```python
from build123d import *

# Parameters (mm, degrees)
CROQUIS1_R                      = 1.625
SALIENTE_EXTRUIR1_DEPTH         = 4
CORTAR_EXTRUIR1_START           = -190
CORTAR_EXTRUIR1_DEPTH           = 190
CROQUIS4_R                      = 3.35997123
CORTAR_EXTRUIR2_DEPTH           = 1.8
CORTAR_EXTRUIR2_DRAFT           = -44
CORTAR_EXTRUIR2_PROFILE_2_DEPTH = 1.8
CORTAR_EXTRUIR2_PROFILE_2_DRAFT = -44
CORTAR_EXTRUIR2_PROFILE_3_DEPTH = 1.8
CORTAR_EXTRUIR2_PROFILE_3_DRAFT = -44
CORTAR_EXTRUIR2_PROFILE_4_DEPTH = 1.8
CORTAR_EXTRUIR2_PROFILE_4_DRAFT = -44
CORTAR_EXTRUIR3_DEPTH           = 2
CROQUIS9_W                      = 0.961538462
CROQUIS9_H                      = 7.5
CORTAR_EXTRUIR5_DEPTH           = 1.5


with BuildPart() as part:
    # Croquis1 → Saliente-Extruir1 (new body)
    with BuildSketch(Plane.XY):
        Polygon((-32.320991683, -51.284123552), (-32.320991683, 29.135238548), (157.679008317, 29.135238548), (157.679008317, -51.284123552), (105.737585684, -51.284123552), (105.737585684, -25.284123552), (45.737585684, -25.284123552), (45.737585684, -51.284123552), align=None)
        with Locations((23.679008317, 21.135238548)):
            Circle(CROQUIS1_R, mode=Mode.SUBTRACT)
        with Locations((101.679008317, 21.135238548)):
            Circle(CROQUIS1_R, mode=Mode.SUBTRACT)
        with Locations((-25.720991683, -43.884123552)):
            Circle(CROQUIS1_R, mode=Mode.SUBTRACT)
        with Locations((151.079008317, -44.084123552)):
            Circle(CROQUIS1_R, mode=Mode.SUBTRACT)
    extrude(amount=SALIENTE_EXTRUIR1_DEPTH)

    # Croquis3 → Cortar-Extruir1 (cut)
    with BuildSketch(Plane(origin=(157.679008317, 0, 0), x_dir=(0, 0, -1), z_dir=(1, 0, 0)).offset(CORTAR_EXTRUIR1_START)):
        Polygon((-4, 29.135238548), (0, 29.135238548), (-4, 27.880003721), align=None)
    extrude(amount=CORTAR_EXTRUIR1_DEPTH, mode=Mode.SUBTRACT)


with BuildPart() as cortar_extruir2_tool:
    # Croquis4 → Cortar-Extruir2 (with draft: the straight prism first)
    with BuildSketch(Plane.XY.offset(4)):
        with Locations((23.679008317, 21.135238548)):
            Circle(CROQUIS4_R)
    extrude(amount=-CORTAR_EXTRUIR2_DEPTH)
    # Cortar-Extruir2: the draft: its side faces are tilted about the plane it starts from
    cortar_extruir2_sides = [cortar_extruir2_tool.faces().sort_by_distance(p)[0] for p in [
        (20.319037087, 21.135238548, 3.1),
    ]]
    draft(cortar_extruir2_sides, Plane.XY.offset(4), CORTAR_EXTRUIR2_DRAFT)


with BuildPart() as part_1:
    add(part.part)

    # Cortar-Extruir2: cut by cortar_extruir2_tool
    add(cortar_extruir2_tool.part, mode=Mode.SUBTRACT)


with BuildPart() as cortar_extruir2_profile_2_tool:
    # Croquis4 → Cortar-Extruir2 profile 2 (with draft: the straight prism first)
    with BuildSketch(Plane.XY.offset(4)):
        with Locations((101.679008317, 21.135238548)):
            Circle(CROQUIS4_R)
    extrude(amount=-CORTAR_EXTRUIR2_PROFILE_2_DEPTH)
    # Cortar-Extruir2 profile 2: the draft: its side faces are tilted about the plane it starts from
    cortar_extruir2_profile_2_sides = [cortar_extruir2_profile_2_tool.faces().sort_by_distance(p)[0] for p in [
        (98.319037087, 21.135238548, 3.1),
    ]]
    draft(cortar_extruir2_profile_2_sides, Plane.XY.offset(4), CORTAR_EXTRUIR2_PROFILE_2_DRAFT)


with BuildPart() as part_2:
    add(part_1.part)

    # Cortar-Extruir2 profile 2: cut by cortar_extruir2_profile_2_tool
    add(cortar_extruir2_profile_2_tool.part, mode=Mode.SUBTRACT)


with BuildPart() as cortar_extruir2_profile_3_tool:
    # Croquis4 → Cortar-Extruir2 profile 3 (with draft: the straight prism first)
    with BuildSketch(Plane.XY.offset(4)):
        with Locations((-25.720991683, -43.884123552)):
            Circle(CROQUIS4_R)
    extrude(amount=-CORTAR_EXTRUIR2_PROFILE_3_DEPTH)
    # Cortar-Extruir2 profile 3: the draft: its side faces are tilted about the plane it starts from
    cortar_extruir2_profile_3_sides = [cortar_extruir2_profile_3_tool.faces().sort_by_distance(p)[0] for p in [
        (-29.080962913, -43.884123552, 3.1),
    ]]
    draft(cortar_extruir2_profile_3_sides, Plane.XY.offset(4), CORTAR_EXTRUIR2_PROFILE_3_DRAFT)


with BuildPart() as part_3:
    add(part_2.part)

    # Cortar-Extruir2 profile 3: cut by cortar_extruir2_profile_3_tool
    add(cortar_extruir2_profile_3_tool.part, mode=Mode.SUBTRACT)


with BuildPart() as cortar_extruir2_profile_4_tool:
    # Croquis4 → Cortar-Extruir2 profile 4 (with draft: the straight prism first)
    with BuildSketch(Plane.XY.offset(4)):
        with Locations((151.079008317, -44.084123552)):
            Circle(CROQUIS4_R)
    extrude(amount=-CORTAR_EXTRUIR2_PROFILE_4_DEPTH)
    # Cortar-Extruir2 profile 4: the draft: its side faces are tilted about the plane it starts from
    cortar_extruir2_profile_4_sides = [cortar_extruir2_profile_4_tool.faces().sort_by_distance(p)[0] for p in [
        (147.719037087, -44.084123552, 3.1),
    ]]
    draft(cortar_extruir2_profile_4_sides, Plane.XY.offset(4), CORTAR_EXTRUIR2_PROFILE_4_DRAFT)


with BuildPart() as part_4:
    add(part_3.part)

    # Cortar-Extruir2 profile 4: cut by cortar_extruir2_profile_4_tool
    add(cortar_extruir2_profile_4_tool.part, mode=Mode.SUBTRACT)

    # Croquis6 → Cortar-Extruir3 (cut)
    with BuildSketch(Plane.XY.offset(4)):
        Polygon((16.032465101, -18.974654774), (-1.066430914, -18.974654774), (-6.350280368, -35.236671251), (-11.634129822, -18.974654774), (-28.733025837, -18.974654774), (-14.899728375, -8.924175866), (-20.183577829, 7.337840611), (-6.350280368, -2.712638297), (7.483017094, 7.337840611), (2.19916764, -8.924175866), align=None)
        Polygon((109.325551533, -18.974654774), (126.424447548, -18.974654774), (131.708297002, -35.236671251), (136.992146456, -18.974654774), (154.091042471, -18.974654774), (140.25774501, -8.924175866), (145.541594464, 7.337840611), (131.708297002, -2.712638297), (117.874999541, 7.337840611), (123.158848995, -8.924175866), align=None)
    extrude(amount=-CORTAR_EXTRUIR3_DEPTH, mode=Mode.SUBTRACT)

    # Croquis9 → Cortar-Extruir5 (cut)
    # profile 1 of 7: a face of its own
    with BuildSketch(Plane.XY.offset(4)):
        Polygon((84.938623702, -0.162159389), (83.97708524, -0.162159389), (83.97708524, 2.546674746), (80.24661649, -0.162159389), (78.832854471, -0.162159389), (83.464765529, 3.203225226), (78.448239086, 7.337840611), (79.771856875, 7.337840611), (83.97708524, 3.871794938), (83.97708524, 7.337840611), (84.938623702, 7.337840611), align=None)
    # profile 2 of 7: a face of its own
    with BuildSketch(Plane.XY.offset(4)):
        Polygon((73.111700625, -0.162159389), (68.688623702, 7.337840611), (69.747818413, 7.337840611), (71.166087644, 4.933994457), (75.309717452, 4.933994457), (76.759537163, 7.337840611), (77.823239086, 7.337840611), (73.304008317, -0.162159389), align=None)
        Polygon((73.21536649, 1.457431957), (74.846977067, 4.164763688), (71.618311202, 4.164763688), align=None, mode=Mode.SUBTRACT)
    # profile 3 of 7: a face of its own
    with BuildSketch(Plane.XY.offset(4)):
        with Locations((66.861700625, 3.587840611)):
            Rectangle(CROQUIS9_W, CROQUIS9_H)
    # profile 4 of 7: a face of its own
    with BuildSketch(Plane.XY.offset(4)):
        with BuildLine():
            Line((64.361700625, -0.162159389), (62.432614086, -0.162159389))
            add(Edge.make_bspline(
                [(62.432614086, -0.162159389), (62.303407857, -0.161829936), (62.056004322, -0.161199101), (61.701380518, -0.157593434), (61.379408986, -0.147395372), (61.089802811, -0.138594846), (60.832957985, -0.122524062), (60.608382947, -0.107262614), (60.416359573, -0.087004293), (60.299642276, -0.06843303), (60.24661649, -0.059995928)],
                knots=[0, 0, 0, 0, 1.415751681, 2.71087525, 3.885633551, 4.945392006, 5.885335126, 6.705178082, 7.411750013, 8, 8, 8, 8], degree=3))
            add(Edge.make_bspline(
                [(60.24661649, -0.059995928), (60.176287708, -0.046434609), (60.037576928, -0.019687366), (59.836939759, 0.036257843), (59.646354736, 0.102761484), (59.465191207, 0.179124214), (59.294103688, 0.267862518), (59.132735961, 0.367086444), (58.982105619, 0.477181944), (58.841971811, 0.596786711), (58.716597542, 0.726930123), (58.605911754, 0.864303479), (58.511163617, 1.009066491), (58.437601574, 1.163087556), (58.375263981, 1.322066158), (58.333771964, 1.489710459), (58.309818392, 1.664567276), (58.305961545, 1.783379506), (58.304008317, 1.843549746)],
                knots=[0, 0, 0, 0, 1.157691968, 2.283337632, 3.364020569, 4.419814557, 5.459210511, 6.477190408, 7.479723838, 8.473058916, 9.452300592, 10.396950777, 11.322316779, 12.24213949, 13.151964026, 14.078922895, 15.027106307, 16, 16, 16, 16], degree=3))
            add(Edge.make_bspline(
                [(58.304008317, 1.843549746), (58.305091786, 1.894193695), (58.307233563, 1.994305563), (58.326423676, 2.141861151), (58.353980579, 2.284876692), (58.39549308, 2.422930299), (58.44745429, 2.556502857), (58.513219778, 2.685284656), (58.589509979, 2.809405247), (58.676822774, 2.929058118), (58.776602841, 3.04093505), (58.884566714, 3.148428384), (59.003880288, 3.24768771), (59.133254395, 3.339146066), (59.272547378, 3.423510414), (59.421274842, 3.50192944), (59.580656173, 3.571958158), (59.750424189, 3.636018975), (59.934268605, 3.69139676), (60.133100327, 3.741243648), (60.349126643, 3.780614055), (60.580514781, 3.815583328), (60.829148914, 3.842258394), (61.094233729, 3.861356634), (61.375810546, 3.873582923), (61.568718995, 3.875378875), (61.667890529, 3.876302149)],
                knots=[0, 0, 0, 0, 0.82629536, 1.63340285, 2.425382263, 3.201336329, 3.983124717, 4.761829792, 5.558184815, 6.35935043, 7.176046838, 8.002665633, 8.844186878, 9.706107795, 10.586553567, 11.500699361, 12.448580803, 13.426410186, 14.460764388, 15.580971395, 16.77061285, 18.043484787, 19.400318222, 20.851143476, 22.381216936, 24, 24, 24, 24], degree=3))
            Line((61.667890529, 3.876302149), (58.207854471, 7.337840611))
            Line((58.207854471, 7.337840611), (59.430811202, 7.337840611))
            Line((59.430811202, 7.337840611), (62.890847259, 3.876302149))
            Line((62.890847259, 3.876302149), (63.400162163, 3.876302149))
            Line((63.400162163, 3.876302149), (63.400162163, 7.337840611))
            Line((63.400162163, 7.337840611), (64.361700625, 7.337840611))
            Line((64.361700625, 7.337840611), (64.361700625, -0.162159389))
        make_face()
        with BuildLine():
            Line((63.400162163, 0.60707138), (63.400162163, 3.10707138))
            Line((63.400162163, 3.10707138), (61.712962644, 3.117588207))
            add(Edge.make_bspline(
                [(61.712962644, 3.117588207), (61.6338262, 3.117624593), (61.48102171, 3.11769485), (61.260170178, 3.109105998), (61.055229731, 3.099416115), (60.865838556, 3.084387818), (60.692378793, 3.065434605), (60.534983254, 3.041372826), (60.393457337, 3.013276714), (60.228708832, 2.970150308), (60.04308286, 2.905086825), (59.845073139, 2.802592369), (59.671455393, 2.679607959), (59.526919773, 2.535743204), (59.408781872, 2.378204093), (59.32775206, 2.207226521), (59.274453943, 2.028014983), (59.268539248, 1.904525416), (59.265546779, 1.842047342)],
                knots=[0, 0, 0, 0, 1.231241804, 2.377403736, 3.438588451, 4.423532574, 5.333122879, 6.153078988, 6.900388758, 7.57703744, 8.802049324, 9.952204265, 11.035615897, 12.099087035, 13.113730954, 14.082638441, 15.029933775, 16, 16, 16, 16], degree=3))
            add(Edge.make_bspline(
                [(59.265546779, 1.842047342), (59.268716736, 1.78162656), (59.275033974, 1.661217199), (59.326660493, 1.485205192), (59.413536844, 1.319765548), (59.52862314, 1.163619228), (59.673346138, 1.024962204), (59.840039394, 0.905484395), (60.027181277, 0.807486158), (60.199202974, 0.742600317), (60.354080103, 0.704099078), (60.489215667, 0.676455153), (60.642999865, 0.656896215), (60.81430402, 0.638812614), (61.003643568, 0.623698235), (61.210563803, 0.613598768), (61.435480972, 0.607489486), (61.59126372, 0.607214564), (61.67239774, 0.60707138)],
                knots=[0, 0, 0, 0, 0.958272772, 1.909690835, 2.884192254, 3.91323511, 4.976135083, 6.053102071, 7.159410583, 8.321911079, 8.96225367, 9.69213132, 10.510867191, 11.422434135, 12.427570329, 13.526393913, 14.711708402, 16, 16, 16, 16], degree=3))
            Line((61.67239774, 0.60707138), (63.400162163, 0.60707138))
        make_face(mode=Mode.SUBTRACT)
    # profile 5 of 7: a face of its own
    with BuildSketch(Plane.XY.offset(4)):
        with Locations((55.804008317, 3.587840611)):
            Rectangle(CROQUIS9_W, CROQUIS9_H)
    # profile 6 of 7: a face of its own
    with BuildSketch(Plane.XY.offset(4)):
        Polygon((53.688623702, 7.337840611), (52.429609279, -0.162159389), (52.088563606, -0.162159389), (48.255931394, 5.991686765), (44.438323221, -0.162159389), (44.085258317, -0.162159389), (42.823239086, 7.337840611), (43.792289567, 7.337840611), (44.698239086, 1.953225226), (48.038082836, 7.337840611), (48.458755913, 7.337840611), (51.813623702, 1.953225226), (52.718070817, 7.337840611), align=None)
    # profile 7 of 7: a face of its own
    with BuildSketch(Plane.XY.offset(4)):
        with Locations((40.611700625, 3.587840611)):
            Rectangle(CROQUIS9_W, CROQUIS9_H)
    extrude(amount=-CORTAR_EXTRUIR5_DEPTH, mode=Mode.SUBTRACT)


solid = part_4.part
```
Read the model definition and answer for the solid it produces. Units are mm, in the model's axes. A direction names the side the tool comes from. Coordinates: 2 decimals unless noted, no trailing zeros. Loops run counter-clockwise (first coordinate to the right, second up) from the corner with the lowest first, then second, coordinate; pieces in that order, holes last.
(1) The part is cut by section B-B (z = 0.95). Determine the outline of the cut face in (x, y) (3 decimals), and give its area (3 significant figures).
Solution:
outline: (-32.321, -51.284) - (45.738, -51.284) - (45.738, -25.284) - (105.738, -25.284) - (105.738, -51.284) - (157.679, -51.284) - (157.679, 28.837) - (-32.321, 28.837) - close; hole circle Ø3.25 at (-25.721, -43.884); hole circle Ø3.25 at (23.679, 21.135); hole circle Ø3.25 at (101.679, 21.135); hole circle Ø3.25 at (151.079, -44.084)
area: 13,600 mm2
(2) Flat-ended cylindrical pins translate along their axes: pin 1 Ø1.6 at (x, z) = (116.5, 3.5) entering from +Y; pin 2 Ø0.5 at (x, z) = (69, 3.5) entering from -Y; pin 3 Ø1 at (x, z) = (11, 2.5) entering from +Y. Find the tip coordinate at first contact, or state that the pin passes through.
Solution:
pin 1: stops at y = 28.29
pin 2: stops at y = -25.28
pin 3: stops at y = 28.51
(3) The part is cut by section C-C (y = -21). Determine the outline of the cut face in (x, z), and give its area (3 significant figures).
Solution:
outline: (-32.32, 0) - (157.68, 0) - (157.68, 4) - (136.33, 4) - (136.33, 2) - (127.08, 2) - (127.08, 4) - (-1.72, 4) - (-1.72, 2) - (-10.98, 2) - (-10.98, 4) - (-32.32, 4) - close
area: 723 mm2
(4) The mould has two halves that part along X. Classify faces 1 (the face through (80.992, 5.242, 3.26)), 2 (the face through (64, -11, 0)), 3 (the face through (50.1, 4.7, 3.3)): released by +X, released by -X, zero draft, split by the parting line, or undercut.
Solution:
face 1: undercut
face 2: zero draft
face 3: undercut
(5) Consider line 1 along X through (y, z) = (-12, 2.1); line 2 along X through (y, z) = (-8, 2.1); line 3 along X through (y, z) = (-26.5, 1.8). Determine where each line is inside the solid, lowest interval first.
Solution:
line 1: x = -32.32 to -19.13, 6.43 to 118.93, 144.49 to 157.68
line 2: x = -32.32 to -15.2, 2.5 to 122.86, 140.56 to 157.68
line 3: x = -32.32 to 45.74, 105.74 to 157.68
(6) The part is cut by section A-A (y = -33.5). Determine the outline of the cut face in (x, z).
Solution:
outline: (-32.32, 0) - (45.74, 0) - (45.74, 4) - (-5.79, 4) - (-5.79, 2) - (-6.91, 2) - (-6.91, 4) - (-32.32, 4) - close; (105.74, 0) - (157.68, 0) - (157.68, 4) - (132.27, 4) - (132.27, 2) - (131.14, 2) - (131.14, 4) - (105.74, 4) - close
(7) A tool of negligible diameter and unlimited length cuts with its end or side. For faces 4 (the face through (103.23, 21.62, 1.09)), 5 (the face through (4.878, -0.679, 3.014)), from which of +Z, -Z, +X, -X, +Y, -Y can it reach the whole face along a straight path? Write none if from no direction.
Solution:
face 4: +Z, -Z
face 5: +Z
